from build123d import *
from OCP.BRepFilletAPI import BRepFilletAPI_MakeChamfer

# Parameters (mm, degrees)
ESQUISSE1_W                  = 28
ESQUISSE1_H                  = 32
BOSS_EXTRU_1_DEPTH           = 7.15
BOSS_EXTRU_2_DEPTH           = 6
CHANFREIN1_SIZE              = 6
ENL_V_MAT_EXTRU_1_DEPTH      = 6
CHANFREIN1_OF_SYM_TRIE1_SIZE = 6
CONG_1_R                     = 1
ESQUISSE4_R                  = 5.25
BOSS_EXTRU_3_DEPTH           = 1
CHANFREIN2_SIZE2             = 1.191753593
CHANFREIN2_SIZE              = 1
ESQUISSE5_R                  = 2.4
BOSS_EXTRU_4_DEPTH           = 3.9
CHANFREIN3_SIZE              = 1
CHANFREIN3_SIZE2             = 1.191753593
ESQUISSE6_W                  = 7.5
ESQUISSE6_H                  = 5
BOSS_EXTRU_5_DEPTH           = 6
CHANFREIN4_SIZE              = 6
CHANFREIN4_SIZE_2            = 1.057961884


with BuildPart() as part:
    # Esquisse1 → Boss.-Extru.1 (new, symmetric)
    with BuildSketch(Plane.XY):
        Rectangle(ESQUISSE1_W, ESQUISSE1_H)
    extrude(amount=BOSS_EXTRU_1_DEPTH, both=True)

    # Esquisse2 → Boss.-Extru.2 (add)
    with BuildSketch(Plane.ZY.offset(14)):
        Polygon((5.95, 14.5), (7.15, 14.5), (7.15, 6.5), (5.366521974, 6.5), (-5.315928015, 6.5), (-7.15, 6.5), (-7.15, 14.5), (-5.95, 14.5), (-5.95, 8.5), (5.95, 8.5), align=None)
    boss_extru_2 = extrude(amount=BOSS_EXTRU_2_DEPTH)

    # Chanfrein1
    chanfrein1_edges = [part.edges().sort_by_distance(p)[0] for p in [
        (-20, 14.5, 6.55),
        (-20, 14.5, -6.55),
    ]]
    chamfer(chanfrein1_edges, length=CHANFREIN1_SIZE - 0.0001)  # a hair under: the kernel refuses the full size

    # Esquisse3 → Enlèv. mat.-Extru.1 (cut)
    with BuildSketch(Plane(origin=(0, 8.5, 0), x_dir=(1, 0, 0), z_dir=(0, 1, 0))):
        with BuildLine():
            Line((-20, 1), (-19.115549442, 1))
            ThreePointArc((-19.115549442, 1), (-15.6, 0), (-19.115549442, -1))
            Line((-19.115549442, -1), (-20, -1))
            Line((-20, -1), (-20, 1))
        make_face()
    enl_v_mat_extru_1 = extrude(amount=-ENL_V_MAT_EXTRU_1_DEPTH, mode=Mode.SUBTRACT)

    # Symétrie1: Boss.-Extru.2, Enlèv. mat.-Extru.1 across plane
    add(boss_extru_2.mirror(Plane(origin=(0, 0, 0), x_dir=(0, 0, 1), z_dir=(1, 0, 0))))
    add(enl_v_mat_extru_1.mirror(Plane(origin=(0, 0, 0), x_dir=(0, 0, 1), z_dir=(1, 0, 0))), mode=Mode.SUBTRACT)

    # Chanfrein1 of Symétrie1
    chanfrein1_of_sym_trie1_edges = [part.edges().sort_by_distance(p)[0] for p in [
        (20, 14.5, 6.55),
        (20, 14.5, -6.55),
    ]]
    chamfer(chanfrein1_of_sym_trie1_edges, length=CHANFREIN1_OF_SYM_TRIE1_SIZE - 0.0001)  # a hair under: the kernel refuses the full size

    # Congé1
    cong_1_edges = [part.edges().sort_by_distance(p)[0] for p in [
        (-14, -16, 0),
        (-14, -4.75, -7.15),
        (-14, -4.75, 7.15),
        (14, -4.75, -7.15),
        (14, -4.75, 7.15),
        (0, -16, -7.15),
        (0, -16, 7.15),
        (14, -16, 0),
    ]]
    fillet(cong_1_edges, radius=CONG_1_R)

    # Esquisse4 → Boss.-Extru.3 (add)
    with BuildSketch(Plane(origin=(0, 16, 0), x_dir=(1, 0, 0), z_dir=(0, 1, 0))):
        with Locations(Location((-7.5, 0, 0), (0, 0, 90))):
            Circle(ESQUISSE4_R)
    extrude(amount=BOSS_EXTRU_3_DEPTH)

    # Chanfrein2
    chanfrein2_edges = [part.edges().sort_by_distance(p)[0] for p in [
        (-7.5, 17, 5.25),
    ]]
    chanfrein2_side = [part.faces().sort_by_distance(p)[0] for p in [
        (-7.5, 16.98, 5.25),
    ]]
    chamfer(chanfrein2_edges, length=CHANFREIN2_SIZE - 0.0001, length2=CHANFREIN2_SIZE2 - 0.0001, reference=chanfrein2_side[0])  # a hair under: the kernel refuses the full size

    # Esquisse5 → Boss.-Extru.4 (add)
    with BuildSketch(Plane(origin=(0, 17, 0), x_dir=(1, 0, 0), z_dir=(0, 1, 0))):
        with Locations(Location((-7.5, 0, 0), (0, 0, 270))):
            Circle(ESQUISSE5_R)
    extrude(amount=BOSS_EXTRU_4_DEPTH)

    # Chanfrein3
    chanfrein3_edges = [part.edges().sort_by_distance(p)[0] for p in [
        (14, 16, 0),
        (0, 16, -7.15),
        (0, 16, 7.15),
        (-14, 16, 0),
    ]]
    chanfrein3_side = [part.faces().sort_by_distance(p)[0] for p in [
        (2.069489218, 16, 0),
    ]]
    chamfer(chanfrein3_edges, length=CHANFREIN3_SIZE, length2=CHANFREIN3_SIZE2, reference=chanfrein3_side[0])

    # Esquisse6 → Boss.-Extru.5 (add)
    with BuildSketch(Plane.ZY.offset(14)):
        with Locations((-0.508404359, -7)):
            Rectangle(ESQUISSE6_W, ESQUISSE6_H)
    extrude(amount=BOSS_EXTRU_5_DEPTH)

    # Chanfrein4
    chanfrein4_edges_1 = [part.edges().sort_by_distance(p)[0] for p in [
        (-20, -7, -4.258404359),
    ]]
    chanfrein4_side_1 = [part.faces().sort_by_distance(p)[0] for p in [
        (-19.978840762, -7, -4.258404359),
    ]]
    chanfrein4_edges_2 = [part.edges().sort_by_distance(p)[0] for p in [
        (-20, -9.5, -0.508404359),
    ]]
    chanfrein4_side_2 = [part.faces().sort_by_distance(p)[0] for p in [
        (-19.978840762, -9.5, -0.508404359),
    ]]
    chanfrein4_edges_3 = [part.edges().sort_by_distance(p)[0] for p in [
        (-20, -7, 3.241595641),
    ]]
    chanfrein4_side_3 = [part.faces().sort_by_distance(p)[0] for p in [
        (-19.978840762, -7, 3.241595641),
    ]]
    chanfrein4_edges_4 = [part.edges().sort_by_distance(p)[0] for p in [
        (-20, -4.5, -0.508404359),
    ]]
    chanfrein4_side_4 = [part.faces().sort_by_distance(p)[0] for p in [
        (-19.978840762, -4.5, -0.508404359),
    ]]
    chanfrein4 = BRepFilletAPI_MakeChamfer(part.part.solid().wrapped)
    for e in chanfrein4_edges_1:
        chanfrein4.Add(CHANFREIN4_SIZE - 0.0001, CHANFREIN4_SIZE_2 - 0.0001, e.wrapped, chanfrein4_side_1[0].wrapped)
    for e in chanfrein4_edges_2:
        chanfrein4.Add(CHANFREIN4_SIZE - 0.0001, CHANFREIN4_SIZE_2 - 0.0001, e.wrapped, chanfrein4_side_2[0].wrapped)
    for e in chanfrein4_edges_3:
        chanfrein4.Add(CHANFREIN4_SIZE - 0.0001, CHANFREIN4_SIZE_2 - 0.0001, e.wrapped, chanfrein4_side_3[0].wrapped)
    for e in chanfrein4_edges_4:
        chanfrein4.Add(CHANFREIN4_SIZE - 0.0001, CHANFREIN4_SIZE_2 - 0.0001, e.wrapped, chanfrein4_side_4[0].wrapped)
    add(Compound.cast(chanfrein4.Shape()), mode=Mode.REPLACE)  # a hair under: the kernel refuses the full size


solid = part.part
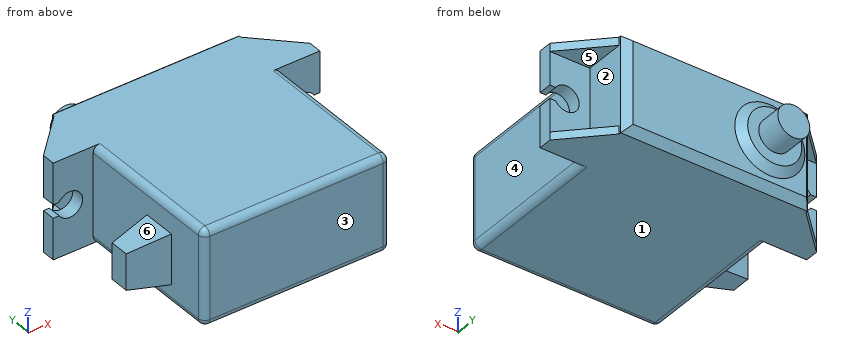
For this review, take the finished solid that the model builds, in its own axes (mm). Face numbers are marked on the shaded views. A direction names the side the tool comes from. Round coordinates to 2 decimals unless told otherwise and drop trailing zeros. Write each loop counter-clockwise with the first axis right and the second up, starting at its lowest first coordinate (ties: lowest second). Pieces come first, ordered by that corner, then holes. Notation, with made-up numbers: (29.25, -16) - (38.25, -16) arc R22 ccw to (38.25, 7) - close; hole circle Ø9 at (-4.5, -27.5). An arc over 180 degrees is marked (long way). Write item = value, one per line. Start each with the question number.
1. For the marked faces 4, 5 and 6, list the 3-axis set-ups (+Z, -Z, +X, -X, +Y, -Y) from which the entire face can be reached by the end or side of a thin tool; tool diameter is ignored.
2. Consider section A-A on x = 17.5. State the section outline as (y, z) points, plus the area to 3 significant figures.
3. Wall thickness on L1, parallel to Z at x = 16, y = 9; L2, parallel to Z at x = 17.5, y = 6.9; L3, parallel to Y at x = 9, z = -4.25: over which ranges is each line inside the solid? List them lowest first.
4. For pin 1 Ø7 at (y, z) = (12.5, -1.5) entering from -X; pin 2 Ø6 at (y, z) = (-3, 1.5) entering from -X; pin 3 Ø5.5 at (x, z) = (-16.5, 2.5) entering from -Y; pin 4 Ø2 at (x, z) = (-1, -3.5) entering from +Y, all flat-tipped, find the tip position at first contact; note any pin that passes through.
5. Consider section B-B on x = -17.5. State the section outline as (y, z) points, plus the area to 3 significant figures.
6. Consider section D-D on x = 1. State the section outline as (y, z) points.
7. Draft analysis for pull direction Z (two halves, no side actions). For the marked faces 1, 2 and 3, state which applies: released by +Z, released by -Z, zero draft, split by the parting line, or undercut.
8. Consider section C-C on y = -11. State the section outline as (x, z) points.
Evaluation:
q1.face_4 = +Z, -Z, +X, -Y
q1.face_5 = +X, +Y
q1.face_6 = +Z, -X, -Y
q2.outline = (6.5, -7.15) - (11, -7.15) - (11, -5.95) - (8.5, -5.95) - (8.5, -1.9) - (6.5, -1.9) - close; (6.5, 1.9) - (8.5, 1.9) - (8.5, 5.95) - (11, 5.95) - (11, 7.15) - (6.5, 7.15) - close
q2.area = 27.0 mm2
q3.L1 = -7.15 to -5.95, 5.95 to 7.15
q3.L2 = -7.15 to -1.9, 1.9 to 7.15
q3.L3 = -16 to 16
q4.pin_1 = -14
q4.pin_2 = -20
q4.pin_3 = -15.66
q4.pin_4 = 16
q5.outline = (-8.88, -3.64) - (-5.12, -3.64) - (-5.12, 2.62) - (-8.88, 2.62) - close; (6.5, -7.15) - (11, -7.15) - (11, -5.95) - (8.5, -5.95) - (8.5, -1.9) - (6.5, -1.9) - close; (6.5, 1.9) - (8.5, 1.9) - (8.5, 5.95) - (11, 5.95) - (11, 7.15) - (6.5, 7.15) - close
q5.area = 50.6 mm2
q6.outline = (-16, -6.15) arc R1 ccw to (-15, -7.15) - (14.81, -7.15) - (16, -6.15) - (16, 6.15) - (14.81, 7.15) - (-15, 7.15) arc R1 ccw to (-16, 6.15) - close
q7.face_1 = released by -Z
q7.face_2 = undercut
q7.face_3 = zero draft
q8.outline = (-14, -6.15) arc R1 ccw to (-13, -7.15) - (13, -7.15) arc R1 ccw to (14, -6.15) - (14, 6.15) arc R1 ccw to (13, 7.15) - (-13, 7.15) arc R1 ccw to (-14, 6.15) - close
